```python
from build123d import *
from OCP.BRepFilletAPI import BRepFilletAPI_MakeChamfer

# Parameters (mm, degrees)
DODANIE_WYCI_GNI_CIE1_DEPTH   = 15
DODANIE_WYCI_GNI_CIE1_2_DEPTH = 15
SZKIC1_3_W                    = 70
SZKIC1_3_H                    = 6.5
DODANIE_WYCI_GNI_CIE2_DEPTH   = 7
SZKIC2_R                      = 9.35
WYTNIJ_WYCI_GNI_CIE1_DEPTH    = 70
DODANIE_WYCI_GNI_CIE3_DEPTH   = 0.3
SFAZOWANIE1_SIZE              = 7
SFAZOWANIE1_SIZE2             = 3.88016336
WYTNIJ_WYCI_GNI_CIE2_REACH    = 82.607
SZKIC4_W                      = 4
SZKIC4_H                      = 0.2
SZKIC4_3_W                    = 4
SZKIC4_3_H                    = 7.8
DODANIE_WYCI_GNI_CIE4_DEPTH   = 0.6
ZAOKR_GLENIE1_R               = 1


with BuildPart() as part:
    # Szkic1 → Dodanie-wyci_gni_cie1 (new body)
    with BuildSketch(Plane(origin=(0, 0, 0), x_dir=(1, 0, 0), z_dir=(0, 1, 0))):
        Polygon((-38.5, -2), (-38.5, -10.5), (-35, -10.5), (-35, 10.5), (-38.5, 10.5), (-38.5, 2), (-36.5, 2), (-36.5, -2), align=None)
    extrude(amount=DODANIE_WYCI_GNI_CIE1_DEPTH)



with BuildPart() as body_2:
    # Szkic1 → Dodanie-wyci_gni_cie1 2 (new body)
    with BuildSketch(Plane(origin=(0, 0, 0), x_dir=(1, 0, 0), z_dir=(0, 1, 0))):
        Polygon((35, 10.5), (35, -10.5), (38.5, -10.5), (38.5, -2), (36.5, -2), (36.5, 2), (38.5, 2), (38.5, 10.5), align=None)
    extrude(amount=DODANIE_WYCI_GNI_CIE1_2_DEPTH)


with BuildPart() as part_1:
    add(part.part)

    add(body_2.part)  # Dodanie-wyci_gni_cie2 merges body 2
    # Szkic1_3 → Dodanie-wyci_gni_cie2 (add)
    with BuildSketch(Plane(origin=(0, 0, 0), x_dir=(1, 0, 0), z_dir=(0, 1, 0))):
        with Locations((0, -7.25)):
            Rectangle(SZKIC1_3_W, SZKIC1_3_H)
        with Locations((0, 7.25)):
            Rectangle(SZKIC1_3_W, SZKIC1_3_H)
    extrude(amount=DODANIE_WYCI_GNI_CIE2_DEPTH)

    # Szkic2 → Wytnij-wyci_gni_cie1 (cut)
    with BuildSketch(Plane(origin=(-35, 0, 0), x_dir=(0, 0, -1), z_dir=(1, 0, 0))):
        with Locations((0, 8.451183349)):
            Circle(SZKIC2_R)
    extrude(amount=WYTNIJ_WYCI_GNI_CIE1_DEPTH, mode=Mode.SUBTRACT)

    # Szkic3 → Dodanie-wyci_gni_cie3 (add)
    with BuildSketch(Plane(origin=(0, 0, 0), x_dir=(1, 0, 0), z_dir=(0, 1, 0))):
        with BuildLine():
            Line((-36.5, 0), (-36.5, 1.9))
            Line((-36.5, 1.9), (-39.5, 1.9))
            Line((-39.5, 1.9), (-39.5, 3))
            Line((-39.5, 3), (-43.5, 3))
            Line((-43.5, 3), (-43.5, 0))
            Line((-43.5, 0), (-42.7, 0))
            ThreePointArc((-42.7, 0), (-42.641421356, 0.141421356), (-42.5, 0.2))
            Line((-42.5, 0.2), (-41.5, 0.2))
            ThreePointArc((-41.5, 0.2), (-41.358578644, 0.141421356), (-41.3, 0))
            Line((-41.3, 0), (-36.5, 0))
        make_face()
        with BuildLine():
            Line((-36.5, -1.9), (-36.5, 0))
            Line((-36.5, 0), (-41.3, 0))
            ThreePointArc((-41.3, 0), (-41.358578644, -0.141421356), (-41.5, -0.2))
            Line((-41.5, -0.2), (-42.5, -0.2))
            ThreePointArc((-42.5, -0.2), (-42.641421356, -0.141421356), (-42.7, 0))
            Line((-42.7, 0), (-43.5, 0))
            Line((-43.5, 0), (-43.5, -3))
            Line((-43.5, -3), (-39.5, -3))
            Line((-39.5, -3), (-39.5, -1.9))
            Line((-39.5, -1.9), (-36.5, -1.9))
        make_face()
        with BuildLine():
            Line((41.5, 0.2), (42.5, 0.2))
            ThreePointArc((42.5, 0.2), (42.641421356, 0.141421356), (42.7, 0))
            Line((42.7, 0), (43.5, 0))
            Line((43.5, 0), (43.5, 3))
            Line((43.5, 3), (39.5, 3))
            Line((39.5, 3), (39.5, 1.9))
            Line((39.5, 1.9), (36.5, 1.9))
            Line((36.5, 1.9), (36.5, 0))
            Line((36.5, 0), (41.3, 0))
            ThreePointArc((41.3, 0), (41.358578644, 0.141421356), (41.5, 0.2))
        make_face()
        with BuildLine():
            Line((43.5, 0), (42.7, 0))
            ThreePointArc((42.7, 0), (42.641421356, -0.141421356), (42.5, -0.2))
            Line((42.5, -0.2), (41.5, -0.2))
            ThreePointArc((41.5, -0.2), (41.358578644, -0.141421356), (41.3, 0))
            Line((41.3, 0), (36.5, 0))
            Line((36.5, 0), (36.5, -1.9))
            Line((36.5, -1.9), (39.5, -1.9))
            Line((39.5, -1.9), (39.5, -3))
            Line((39.5, -3), (43.5, -3))
            Line((43.5, -3), (43.5, 0))
        make_face()
    extrude(amount=DODANIE_WYCI_GNI_CIE3_DEPTH)

    # Sfazowanie1: one chamfer whose edges measure the first distance from different faces: ONE call of the kernel's chamfer builder (chamfer() names one face for all edges)
    sfazowanie1_edges_1 = [part_1.edges().sort_by_distance(p)[0] for p in [
        (-36.75, 15, 10.5),
        (36.75, 15, 10.5),
    ]]
    sfazowanie1_side_1 = [part_1.faces().sort_by_distance(p)[0] for p in [
        (0, 4.205882353, 10.5),
    ]]
    sfazowanie1_edges_2 = [part_1.edges().sort_by_distance(p)[0] for p in [
        (-36.75, 15, -10.5),
        (36.75, 15, -10.5),
    ]]
    sfazowanie1_side_2 = [part_1.faces().sort_by_distance(p)[0] for p in [
        (0, 4.205882353, -10.5),
    ]]
    sfazowanie1 = BRepFilletAPI_MakeChamfer(part_1.part.solid().wrapped)
    for e in sfazowanie1_edges_1:
        sfazowanie1.Add(SFAZOWANIE1_SIZE, SFAZOWANIE1_SIZE2, e.wrapped, sfazowanie1_side_1[0].wrapped)  # the first distance lies on this face
    for e in sfazowanie1_edges_2:
        sfazowanie1.Add(SFAZOWANIE1_SIZE, SFAZOWANIE1_SIZE2, e.wrapped, sfazowanie1_side_2[0].wrapped)  # the first distance lies on this face
    add(Compound.cast(sfazowanie1.Shape()), mode=Mode.REPLACE)

    # Szkic4 → Wytnij-wyci_gni_cie2 (cut, up to next)
    with BuildSketch(Plane(origin=(-35, 0, 0), x_dir=(0, 0, -1), z_dir=(1, 0, 0)), mode=Mode.PRIVATE) as wytnij_wyci_gni_cie2_sk1:
        with Locations((0, 14.9)):
            Rectangle(SZKIC4_W, SZKIC4_H)
    wytnij_wyci_gni_cie2_tool1 = extrude(wytnij_wyci_gni_cie2_sk1.sketch, amount=-WYTNIJ_WYCI_GNI_CIE2_REACH, mode=Mode.PRIVATE) & part_1.part
    wytnij_wyci_gni_cie2 = wytnij_wyci_gni_cie2_tool1.solids().sort_by_distance((-35, 14.9, 0))[0]
    add(wytnij_wyci_gni_cie2, mode=Mode.SUBTRACT)

    # Szkic4_3 → Dodanie-wyci_gni_cie4 (add)
    with BuildSketch(Plane(origin=(-35, 0, 0), x_dir=(0, 0, -1), z_dir=(1, 0, 0))):
        with Locations((0, 10.9)):
            Rectangle(SZKIC4_3_W, SZKIC4_3_H)
    dodanie_wyci_gni_cie4 = extrude(amount=DODANIE_WYCI_GNI_CIE4_DEPTH)

    # Lustro1: Wytnij-wyci_gni_cie2, Dodanie-wyci_gni_cie4 across plane
    add(wytnij_wyci_gni_cie2.mirror(Plane(origin=(0, 0, 0), x_dir=(0, 0, 1), z_dir=(1, 0, 0))), mode=Mode.SUBTRACT)
    add(dodanie_wyci_gni_cie4.mirror(Plane(origin=(0, 0, 0), x_dir=(0, 0, 1), z_dir=(1, 0, 0))))

    # Zaokr_glenie1
    # the kernel refuses this fillet: 1 mm, written as the material it takes off along each edge
    with BuildSketch(Plane(origin=(-36.5, 14.8, -2), x_dir=(0, -1, 0), z_dir=(0, 0, 1)), Plane(origin=(-34.4, 14.8, -2), x_dir=(-1, 0, 0), z_dir=(0, 0, 1))) as zaokr_glenie1_piece_1:
        with BuildLine():
            CenterArc((ZAOKR_GLENIE1_R, ZAOKR_GLENIE1_R), ZAOKR_GLENIE1_R, 180, 90)
            Line((0, ZAOKR_GLENIE1_R), (0, 0))
            Line((0, 0), (ZAOKR_GLENIE1_R, 0))
        make_face()
    extrude(amount=4, mode=Mode.SUBTRACT)
    with BuildSketch(Plane(origin=(36.5, 14.8, -2), x_dir=(0, -1, 0), z_dir=(0, 0, 1)), Plane(origin=(34.4, 14.8, -2), x_dir=(1, 0, 0), z_dir=(0, 0, 1))) as zaokr_glenie1_piece_2:
        with BuildLine():
            CenterArc((ZAOKR_GLENIE1_R, -ZAOKR_GLENIE1_R), ZAOKR_GLENIE1_R, 90, 90)
            Line((0, -ZAOKR_GLENIE1_R), (0, 0))
            Line((0, 0), (ZAOKR_GLENIE1_R, 0))
        make_face()
    extrude(amount=4, mode=Mode.SUBTRACT)


solid = part_1.part
```
Can you work these out from the model? Positions are in its coordinate system, mm. A direction names the side the tool comes from. Coordinates: 2 decimals unless noted, no trailing zeros. Loops run counter-clockwise (first coordinate to the right, second up) from the corner with the lowest first, then second, coordinate; pieces in that order, holes last. Notation, with made-up numbers: (-26.5, -6.75) -> (-2.5, -6.75) arc R35 ccw to (-2.5, 30.25) -> close; hole circle Ø1 at (84.25, 76). An arc over 180 degrees is marked (long way). Put each result on its own line as item: value. Start each with the question number.
Q1. I want a section at B-B (x = -10.5). Write out the boundary of the cut face in (y, z).
Q2. I want a section at D-D (y = 2.25). Write out the boundary of the cut face in (x, z), plus the area to 3 significant figures.
Q3. I want a section at C-C (y = 9.25). Write out the boundary of the cut face in (x, z).
Q4. If I drill on line 1 (X direction, y = 12, z = -5.25); line 2 (X direction, y = 12, z = 0.75); line 3 (Z direction, x = 38, y = 13), over which ranges is the centre line in solid material (lowest first)? Write a range as [from, to].
Q5. I'm going to push flat-ended pins straight in: P1, Ø4, axis at x = 36, y = 11, coming from the +Z side; P2, Ø5, axis at y = 5.5, z = 1, coming from the -X side; P3, Ø1.8, axis at x = 39.5, z = 1, coming from the +Y side. Where does each tip first touch, or does it pass through?
Q6. For faces 1 (the face through (34.4, 10, 0)), 2 (the face through (41, 0.3, 0)), 3 (the face through (-41, 0.3, 0)), 4 (the face through (-0.49, 2.8, -7.45)), which set-ups out of +Z, -Z, +X, -X, +Y, -Y let a thin tool reach every point of the face, with its end or its side?
Q7. I want a section at A-A (z = -1). Write out the boundary of the cut face in (x, y), plus the area to 3 significant figures.
Taken from the geometry:
1. outline: (0, -10.5) -> (7, -10.5) -> (7, -9.24) arc R9.35 cw to (0, -4) -> close; (0, 4) arc R9.35 cw to (7, 9.24) -> (7, 10.5) -> (0, 10.5) -> close
2. outline: (-38.5, -10.5) -> (38.5, -10.5) -> (38.5, -2) -> (36.5, -2) -> (36.5, 2) -> (38.5, 2) -> (38.5, 10.5) -> (-38.5, 10.5) -> (-38.5, 2) -> (-36.5, 2) -> (-36.5, -2) -> (-38.5, -2) -> close; hole (-35, -7) -> (35, -7) -> (35, 7) -> (-35, 7) -> close
2. area: 621 mm2
3. outline: (-38.5, -9.81) -> (-35, -9.81) -> (-35, -2) -> (-34.4, -2) -> (-34.4, 2) -> (-35, 2) -> (-35, 9.81) -> (-38.5, 9.81) -> (-38.5, 2) -> (-36.5, 2) -> (-36.5, -2) -> (-38.5, -2) -> close; (34.4, -2) -> (35, -2) -> (35, -9.81) -> (38.5, -9.81) -> (38.5, -2) -> (36.5, -2) -> (36.5, 2) -> (38.5, 2) -> (38.5, 9.81) -> (35, 9.81) -> (35, 2) -> (34.4, 2) -> close
4. line 1: x = [-38.5, -35], [35, 38.5]
4. line 2: x = [-36.5, -34.4], [34.4, 36.5]
4. line 3: z = [-7.73, -2], [2, 7.73]
5. P1: stops at z = 9.95
5. P2: stops at x = -38.5
5. P3: stops at y = 0.3
6. face 1: +Z, -Z, +Y, -Y
6. face 2: +X, +Y
6. face 3: -X, +Y
6. face 4: +Y
7. outline: (-43.5, 0) -> (-35, 0) -> (-35, 7) -> (-34.4, 7) -> (-34.4, 13.8) arc R1 ccw to (-35.4, 14.8) -> (-35.5, 14.8) arc R1 ccw to (-36.5, 13.8) -> (-36.5, 0.3) -> (-43.5, 0.3) -> close; (34.4, 7) -> (35, 7) -> (35, 0) -> (43.5, 0) -> (43.5, 0.3) -> (36.5, 0.3) -> (36.5, 13.8) arc R1 ccw to (35.5, 14.8) -> (35.4, 14.8) arc R1 ccw to (34.4, 13.8) -> close
7. area: 57.1 mm2
